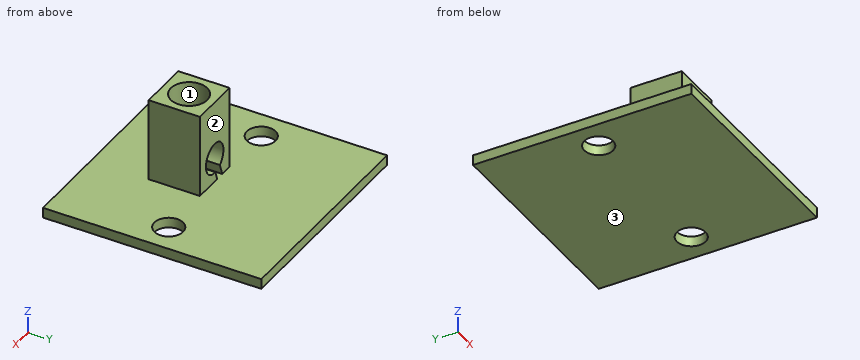
from build123d import *

# Parameters (mm, degrees)
SKETCH1_W           = 34.1
SKETCH1_H           = 34.1
SKETCH1_R           = 2.25
BOSS_EXTRUDE1_DEPTH = 1.6
SKETCH2_W           = 8
SKETCH2_H           = 17
BOSS_EXTRUDE2_DEPTH = 13
SKETCH12_R          = 2.375
CUT_EXTRUDE3_DEPTH  = 18
CUT_EXTRUDE4_DEPTH  = 12
SKETCH14_R          = 2.85
CUT_EXTRUDE9_DEPTH  = 5.7
CUT_EXTRUDE10_REACH = 10.9
SKETCH15_R          = 1.85
SKETCH19_W          = 13
SKETCH19_H          = 9
CUT_EXTRUDE11_DEPTH = 22.05


with BuildPart() as part:
    # Sketch1 → Boss-Extrude1 (new body)
    with BuildSketch(Plane.XY):
        Rectangle(SKETCH1_W, SKETCH1_H)
        with Locations((-12.55, 0)):
            Circle(SKETCH1_R, mode=Mode.SUBTRACT)
        with Locations((12.55, 0)):
            Circle(SKETCH1_R, mode=Mode.SUBTRACT)
    extrude(amount=BOSS_EXTRUDE1_DEPTH)

    # Sketch2 → Boss-Extrude2 (add)
    with BuildSketch(Plane.XY.offset(1.6)):
        with Locations((0, -8.55)):
            Rectangle(SKETCH2_W, SKETCH2_H)
    extrude(amount=BOSS_EXTRUDE2_DEPTH)

    # Sketch12 → Cut-Extrude3 (cut, through all)
    with BuildSketch(Plane(origin=(0, -0.05, 0), x_dir=(1, 0, 0), z_dir=(0, 1, 0))):
        with Locations((0, -5.4)):
            Circle(SKETCH12_R)
    extrude(amount=-CUT_EXTRUDE3_DEPTH, mode=Mode.SUBTRACT)

    # Sketch13 → Cut-Extrude4 (cut)
    with BuildSketch(Plane(origin=(0, -0.05, 0), x_dir=(1, 0, 0), z_dir=(0, 1, 0))):
        Polygon((-1.392084192, -3.475752978), (-2.074802442, -1.6), (-0.691371338, -1.6), (-0.170483785, -3.031126791), align=None)
    extrude(amount=-CUT_EXTRUDE4_DEPTH, mode=Mode.SUBTRACT)

    # Sketch14 → Cut-Extrude9 (cut)
    with BuildSketch(Plane.XY.offset(14.6)):
        with Locations((0, -12.55)):
            Circle(SKETCH14_R)
        with Locations((0, -4.05)):
            Circle(SKETCH14_R)
    extrude(amount=-CUT_EXTRUDE9_DEPTH, mode=Mode.SUBTRACT)

    # Sketch15 → Cut-Extrude10 (cut, up to next)
    with BuildSketch(Plane.XY.offset(8.9), mode=Mode.PRIVATE) as cut_extrude10_sk1:
        with Locations((0, -4.05)):
            Circle(SKETCH15_R)
    cut_extrude10_tool1 = extrude(cut_extrude10_sk1.sketch, amount=-CUT_EXTRUDE10_REACH, mode=Mode.PRIVATE) & part.part
    add(cut_extrude10_tool1.solids().sort_by_distance((0, -4.05, 8.9))[0], mode=Mode.SUBTRACT)
    # Sketch15 → Cut-Extrude10 (cut, up to next)
    with BuildSketch(Plane.XY.offset(8.9), mode=Mode.PRIVATE) as cut_extrude10_sk2:
        with Locations((0, -12.55)):
            Circle(SKETCH15_R)
    cut_extrude10_tool2 = extrude(cut_extrude10_sk2.sketch, amount=-CUT_EXTRUDE10_REACH, mode=Mode.PRIVATE) & part.part
    add(cut_extrude10_tool2.solids().sort_by_distance((0, -12.55, 8.9))[0], mode=Mode.SUBTRACT)

    # Sketch19 → Cut-Extrude11 (cut, through all)
    with BuildSketch(Plane.ZY.offset(4)):
        with Locations((8.1, -12.55)):
            Rectangle(SKETCH19_W, SKETCH19_H)
    extrude(amount=-CUT_EXTRUDE11_DEPTH, mode=Mode.SUBTRACT)


solid = part.part
For this review, take the finished solid that the model builds, in its own axes (mm). Face numbers are marked on the shaded views. Round coordinates to 2 decimals unless told otherwise and drop trailing zeros. Order: outer loops, then holes, each group sorted by start corner. A loop starts at its lowest first (then second) coordinate and runs counter-clockwise, first axis right, second up. Notation, with made-up numbers: M 89.5,24.25 L 109.5,24.25 A21 cw 109.5,60.25 Z; hole C -11,32.5 d9. An arc over 180 degrees is marked long. Use a Markdown table: item, result. Add a question column.
Item 1: Mouldability with a two-part tool opening along Y and no side actions: class the marked faces 1, 2 and 3 as released by +Y, released by -Y, zero draft, split by the parting line, or undercut.
Item 2: Add section A-A, the plane x = 12.55. Give the boundary of the cut face in (y, z).
Item 3: Insertion check: pin 1 (4 mm diameter, centred on x = -6, y = 13, fed in from +Z); pin 2 (4 mm diameter, centred on y = -3, z = 10.5, fed in from -X); pin 3 (2.5 mm diameter, centred on x = -1.5, z = 10.5, fed in from -Y); pin 4 (4 mm diameter, centred on x = 0, z = 5.4, fed in from -Y). Each pin has a flat end and moves straight along its axis. Give the tip position at first contact, or say it passes through.
Item 4: Add section C-C, the plane y = -4.05. Give the boundary of the cut face in (x, z) (3 decimals), then the cut area to 3 significant figures.
Item 5: Add section B-B, the plane z = 10.75. Give the boundary of the cut face in (x, y).
Item 6: Add section D-D, the plane z = 5.25. Give the boundary of the cut face in (x, y), then the cut area to 3 significant figures.
Item 7: To check wall thickness, follow line 1 along Y through (x, z) = (0, 8.55); line 2 along X through (y, z) = (-1.75, 5.4) (3 decimals); line 3 along Y through (x, z) = (12.55, 0.5). State the ranges of each line that lie inside material, in increasing order.
Geometry results:
| question | item | result |
|---|---|---|
| 1 | face 1 | undercut |
| 1 | face 2 | released by +Y |
| 1 | face 3 | zero draft |
| 2 | outline | M -17.05,0 L -2.25,0 L -2.25,1.6 L -17.05,1.6 Z; M 2.25,0 L 17.05,0 L 17.05,1.6 L 2.25,1.6 Z |
| 3 | pin 1 | stops at z = 1.6 |
| 3 | pin 2 | stops at x = -4 |
| 3 | pin 3 | stops at y = -8.05 |
| 3 | pin 4 | passes through |
| 4 | outline | M -17.05,0 L 17.05,0 L 17.05,1.6 L 4,1.6 L 4,14.6 L 2.85,14.6 L 2.85,8.9 L 1.85,8.9 L 1.85,6.889 A2.375 cw -0.17,3.031 L -0.691,1.6 L -2.075,1.6 L -1.392,3.476 A2.375 cw -1.85,6.889 L -1.85,8.9 L -2.85,8.9 L -2.85,14.6 L -4,14.6 L -4,1.6 L -17.05,1.6 Z |
| 4 | area | 101 mm² |
| 5 | outline | M -4,-8.05 L 4,-8.05 L 4,-0.05 L -4,-0.05 Z; hole C 0,-4.05 d5.7 |
| 6 | outline | M -4,-8.05 L -2.37,-8.05 L -2.37,-0.05 L -4,-0.05 Z; M 2.37,-8.05 L 4,-8.05 L 4,-0.05 L 2.37,-0.05 Z |
| 6 | area | 26.1 mm² |
| 7 | line 1 | y = -8.05 to -5.9, -2.2 to -0.05 |
| 7 | line 2 | x = -4 to -2.375, 2.375 to 4 |
| 7 | line 3 | y = -17.05 to -2.25, 2.25 to 17.05 |
